CAD build for the part. Positions are in the model's coordinates, mm. Give positions to 0.01 mm unless a question says otherwise; leave off trailing zeros. Write each loop counter-clockwise with the first axis right and the second up, starting at its lowest first coordinate (ties: lowest second). Pieces come first, ordered by that corner, then holes. Notation, with made-up numbers: (67, 39.5) - (110, 39.5) arc R18 cw to (110, 74.5) - close; hole circle Ø10 at (70, 56). An arc over 180 degrees is marked (long way). Put each result on its own line as item: value. Start each with the question number.
1. Drop a flat-ended pin along its axis: pin 1 (2.5 mm diameter, centred on y = 5.7, z = 39.65, fed in from -X). Give the stop position or say it passes through.
2. Wall check: line 1 (Y direction, x = 7, z = 11); line 2 (Y direction, x = 6.25, z = 183.5). Give the ranges that are in metal, low to high.
3. Cut at A-A on z = 27. List the corners of the cut face in (x, y).
from build123d import *

# Parameters (mm, degrees)
SKETCH_W     = 11.4
SKETCH_H     = 11.4
SKETCH_R     = 1.5
PAD_DEPTH    = 207
SKETCH001_R  = 1.5
POCKET_DEPTH = 11.401


with BuildPart() as part:
    # Sketch → Pad (new body)
    with BuildSketch(Plane.XY):
        with Locations((5.7, 5.7)):
            Rectangle(SKETCH_W, SKETCH_H)
        with Locations((5.7, 5.7)):
            Circle(SKETCH_R, mode=Mode.SUBTRACT)
    extrude(amount=PAD_DEPTH)

    # Sketch001 → Pocket (cut, through all)
    with BuildSketch(Plane.YZ.offset(11.4)):
        with Locations((5.7, 39.65)):
            Circle(SKETCH001_R)
        with Locations((5.7, 31.65)):
            Circle(SKETCH001_R)
        with Locations((5.7, 19)):
            Circle(SKETCH001_R)
        with Locations((5.7, 11)):
            Circle(SKETCH001_R)
        with Locations((5.7, 196)):
            Circle(SKETCH001_R)
        with Locations((5.7, 188)):
            Circle(SKETCH001_R)
    extrude(amount=-POCKET_DEPTH, mode=Mode.SUBTRACT)


solid = part.part
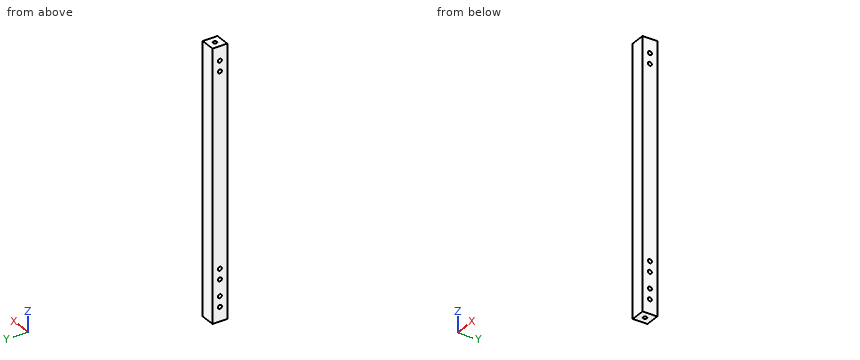
Report:
1. pin 1: passes through
2. line 1: y = 0 to 4.2, 7.2 to 11.4
2. line 2: y = 0 to 4.3, 7.1 to 11.4
3. outline: (0, 0) - (11.4, 0) - (11.4, 11.4) - (0, 11.4) - close; hole circle Ø3 at (5.7, 5.7)
